For this review, use the dimensioned drawing (mm, ordinates from the lowest corner) and the shaded views. A direction names the side the tool comes from. Give positions to 0.01 mm unless a question says otherwise; leave off trailing zeros. Order: outer loops, then holes, each group sorted by start corner. A loop starts at its lowest first (then second) coordinate and runs counter-clockwise, first axis right, second up. Notation, with made-up numbers: (18, -21.5) - (69, -21.5) arc R33 cw to (69, 7.5) - close; hole circle Ø11 at (33, 78). An arc over 180 degrees is marked (long way). Use a Markdown table: item, result. Add a question column.
1) We need section D-D on y = 4.75. Write out the cut boundary in (x, z).
2) Clearance check with flat-ended pins moving along their axes: P1, Ø3, axis at x = 9, z = 1.75, coming from the +Y side; P2, Ø1.5, axis at y = 1, z = 1.5, coming from the -X side; P3, Ø1.4, axis at y = 5.5, z = 3.5, coming from the +X side. State where each tip first meets the part, or that it passes through.
3) We need section C-C on z = 6. Write out the cut boundary in (x, y), then the cut area to 3 significant figures.
4) Machinability: for the marked faces 1, 2 and 3, which of the approach directions +Z, -Z, +X, -X, +Y, -Y give a long, thin tool a straight path to every point of the face, cutting with its end or side? Answer none if there is none.
5) We need section B-B on x = 9.5. Write out the cut boundary in (y, z).
6) Wall thickness on L1, parallel to Z at x = 9, y = 1; L2, parallel to Y at x = 10, z = 7; L3, parallel to X at y = 4, z = 4: over which ranges is each line inside the solid? List them lowest first.
7) Mouldability with a two-part tool opening along Z and no side actions: class the marked faces 4, 5, 6 and 7 as released by +Z, released by -Z, zero draft, split by the parting line, or undercut.
8) We need section A-A on z = 1.75. Write out the cut boundary in (x, y), then the cut area to 3 significant figures.
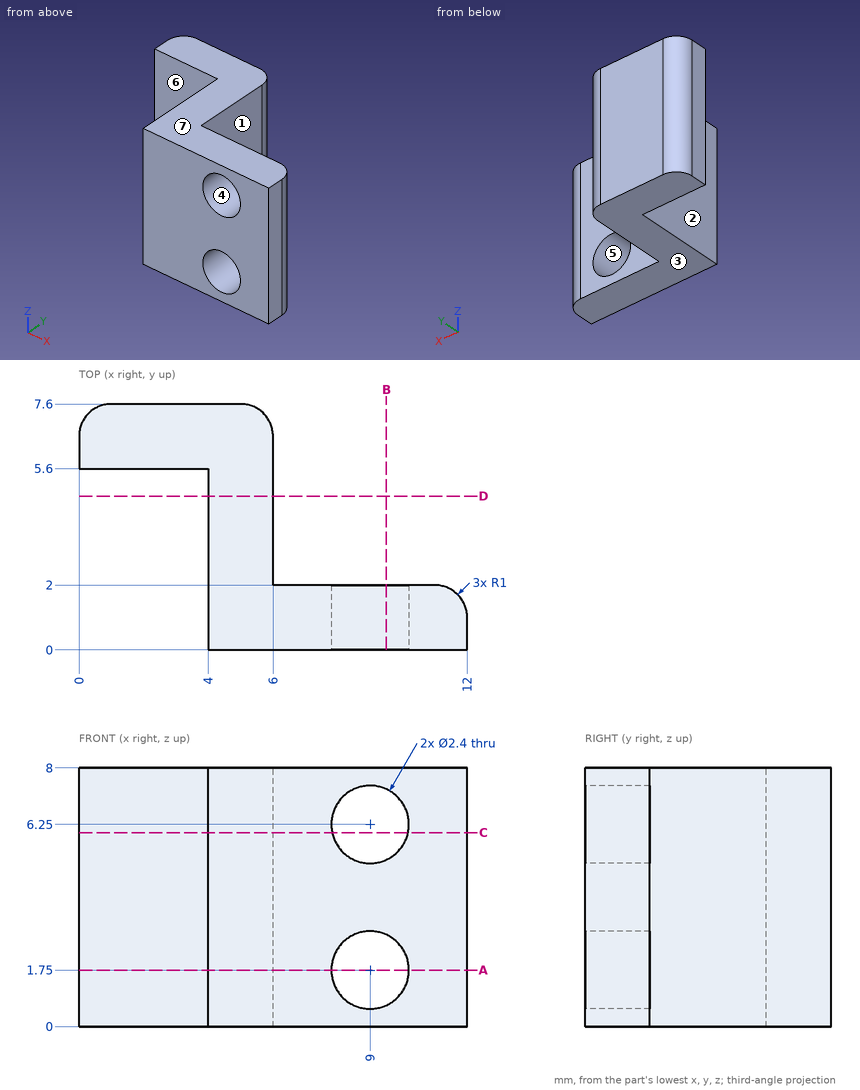
Checked values:
| question | item | result |
|---|---|---|
| 1 | outline | (4, 0) - (6, 0) - (6, 8) - (4, 8) - close |
| 2 | P1 | y = 2 |
| 2 | P2 | x = 4 |
| 2 | P3 | x = 6 |
| 3 | outline | (0, 5.6) - (4, 5.6) - (4, 0) - (7.83, 0) - (7.83, 2) - (6, 2) - (6, 6.6) arc R1 ccw to (5, 7.6) - (1, 7.6) arc R1 ccw to (0, 6.6) - close; (10.17, 0) - (12, 0) - (12, 1) arc R1 ccw to (11, 2) - (10.17, 2) - close |
| 3 | area | 29.9 mm² |
| 4 | face 1 | +Z, -Z, +X, +Y |
| 4 | face 2 | +Z, -Z, -X, -Y |
| 4 | face 3 | -Z, +X, -X, +Y, -Y |
| 5 | outline | (0, 0) - (2, 0) - (2, 0.66) - (0, 0.66) - close; (0, 2.84) - (2, 2.84) - (2, 5.16) - (0, 5.16) - close; (0, 7.34) - (2, 7.34) - (2, 8) - (0, 8) - close |
| 6 | L1 | 0 to 0.55, 2.95 to 5.05, 7.45 to 8 |
| 6 | L2 | 0 to 2 |
| 6 | L3 | 4 to 6 |
| 7 | face 4 | undercut |
| 7 | face 5 | undercut |
| 7 | face 6 | zero draft |
| 7 | face 7 | released by +Z |
| 8 | outline | (0, 5.6) - (4, 5.6) - (4, 0) - (7.8, 0) - (7.8, 2) - (6, 2) - (6, 6.6) arc R1 ccw to (5, 7.6) - (1, 7.6) arc R1 ccw to (0, 6.6) - close; (10.2, 0) - (12, 0) - (12, 1) arc R1 ccw to (11, 2) - (10.2, 2) - close |
| 8 | area | 29.8 mm² |
